```python
from build123d import *

# Parameters (mm, degrees)
SKETCH_1_W          = 100
SKETCH_1_H          = 75
EXTRUDE_1_DEPTH     = 3
SKETCH_2_R          = 2.5
CUT_EXTRUDE_1_DEPTH = 3
SKETCH_3_R          = 2.5
CUT_EXTRUDE_2_DEPTH = 3
EXTRUDE_2_DEPTH     = 3
FILLET_1_R          = 1.5


with BuildPart() as part:
    # 草图1 → 凸台-拉伸1 (new body)
    with BuildSketch(Plane(origin=(0, 0, 0), x_dir=(1, 0, 0), z_dir=(0, 1, 0))):
        Rectangle(SKETCH_1_W, SKETCH_1_H)
    extrude(amount=EXTRUDE_1_DEPTH)

    # 草图2 → 切除-拉伸1 (cut)
    with BuildSketch(Plane(origin=(0, 3, 0), x_dir=(1, 0, 0), z_dir=(0, 1, 0))):
        with Locations(Location((-46.9, 17.87, 0), (0, 0, 270))):
            Circle(SKETCH_2_R)
        with Locations(Location((-46.9, -31.338, 0), (0, 0, 90))):
            Circle(SKETCH_2_R)
        with Locations(Location((40.184, -31.338, 0), (0, 0, 270))):
            Circle(SKETCH_2_R)
        with Locations(Location((40.184, 17.87, 0), (0, 0, 90))):
            Circle(SKETCH_2_R)
    extrude(amount=-CUT_EXTRUDE_1_DEPTH, mode=Mode.SUBTRACT)

    # 草图3 → 切除-拉伸2 (cut)
    with BuildSketch(Plane(origin=(0, 3, 0), x_dir=(1, 0, 0), z_dir=(0, 1, 0))):
        with Locations(Location((-24, 25, 0), (0, 0, 270))):
            Circle(SKETCH_3_R)
        with Locations(Location((24, 25, 0), (0, 0, 90))):
            Circle(SKETCH_3_R)
        with Locations(Location((24, -25, 0), (0, 0, 270))):
            Circle(SKETCH_3_R)
        with Locations(Location((-24, -25, 0), (0, 0, 90))):
            Circle(SKETCH_3_R)
        with Locations(Location((0, 5, 0), (0, 0, 270))):
            Circle(SKETCH_3_R)
        with Locations(Location((0, 15, 0), (0, 0, 270))):
            Circle(SKETCH_3_R)
        with Locations(Location((0, -15, 0), (0, 0, 90))):
            Circle(SKETCH_3_R)
        with Locations(Location((0, -5, 0), (0, 0, 90))):
            Circle(SKETCH_3_R)
        with Locations(Location((10, 5, 0), (0, 0, 270))):
            Circle(SKETCH_3_R)
        with Locations(Location((10, 15, 0), (0, 0, 270))):
            Circle(SKETCH_3_R)
        with Locations(Location((10, -15, 0), (0, 0, 90))):
            Circle(SKETCH_3_R)
        with Locations(Location((10, -5, 0), (0, 0, 90))):
            Circle(SKETCH_3_R)
        with Locations(Location((20, 5, 0), (0, 0, 270))):
            Circle(SKETCH_3_R)
        with Locations(Location((20, 15, 0), (0, 0, 270))):
            Circle(SKETCH_3_R)
        with Locations(Location((20, -15, 0), (0, 0, 90))):
            Circle(SKETCH_3_R)
        with Locations(Location((20, -5, 0), (0, 0, 90))):
            Circle(SKETCH_3_R)
        with Locations(Location((-20, -5, 0), (0, 0, 270))):
            Circle(SKETCH_3_R)
        with Locations(Location((-20, -15, 0), (0, 0, 270))):
            Circle(SKETCH_3_R)
        with Locations(Location((-20, 15, 0), (0, 0, 90))):
            Circle(SKETCH_3_R)
        with Locations(Location((-20, 5, 0), (0, 0, 90))):
            Circle(SKETCH_3_R)
        with Locations(Location((-10, -5, 0), (0, 0, 270))):
            Circle(SKETCH_3_R)
        with Locations(Location((-10, -15, 0), (0, 0, 270))):
            Circle(SKETCH_3_R)
        with Locations(Location((-10, 15, 0), (0, 0, 90))):
            Circle(SKETCH_3_R)
        with Locations(Location((-10, 5, 0), (0, 0, 90))):
            Circle(SKETCH_3_R)
        with BuildLine():
            Line((-31.51322225, 8.5), (-31.51322225, -8.5))
            ThreePointArc((-31.51322225, -8.5), (-36.01322225, -13), (-40.51322225, -8.5))
            Line((-40.51322225, -8.5), (-40.51322225, 8.5))
            ThreePointArc((-40.51322225, 8.5), (-36.01322225, 13), (-31.51322225, 8.5))
        make_face()
        with BuildLine():
            Line((31.51322225, 8.5), (31.51322225, -8.5))
            ThreePointArc((31.51322225, -8.5), (36.01322225, -13), (40.51322225, -8.5))
            Line((40.51322225, -8.5), (40.51322225, 8.5))
            ThreePointArc((40.51322225, 8.5), (36.01322225, 13), (31.51322225, 8.5))
        make_face()
    extrude(amount=-CUT_EXTRUDE_2_DEPTH, mode=Mode.SUBTRACT)

    # 草图4 → 凸台-拉伸2 (add)
    with BuildSketch(Plane(origin=(0, 3, 0), x_dir=(1, 0, 0), z_dir=(0, 1, 0))):
        Polygon((-50, 22.87), (-51.2, 20.296591695), (-51.2, 15.443408305), (-50, 12.87), align=None)
        Polygon((-51.2, -28.911408305), (-50, -26.338), (-50, -36.338), (-51.2, -33.764591695), align=None)
    extrude(amount=-EXTRUDE_2_DEPTH)

    # 圆角1
    # the kernel refuses this fillet: 1.5 mm, written as the material it takes off along each edge
    with BuildSketch(Plane(origin=(50, -3.75, 37.5), x_dir=(0, 0, -1), z_dir=(0, 1, 0)), Plane(origin=(50, -3.75, -37.5), x_dir=(-1, 0, 0), z_dir=(0, 1, 0))) as fillet_1_piece_1:
        with BuildLine():
            CenterArc((FILLET_1_R, FILLET_1_R), FILLET_1_R, 180, 90)
            Line((0, FILLET_1_R), (-FILLET_1_R * 0.02, FILLET_1_R))
            Line((-FILLET_1_R * 0.02, FILLET_1_R), (-FILLET_1_R * 0.02, -FILLET_1_R * 0.02))
            Line((-FILLET_1_R * 0.02, -FILLET_1_R * 0.02), (FILLET_1_R, -FILLET_1_R * 0.02))
            Line((FILLET_1_R, -FILLET_1_R * 0.02), (FILLET_1_R, 0))
        make_face()
    extrude(amount=10.5, mode=Mode.SUBTRACT)
    with BuildSketch(Plane(origin=(-50, -3.653556486, 37.5), x_dir=(1, 0, 0), z_dir=(0, 1, 0))) as fillet_1_piece_2:
        with BuildLine():
            CenterArc((1.461422595, 1.5), FILLET_1_R, 193.02248013, 76.97751987)
            Line((0, 1.162), (-0.029228452, 1.15524))
            ThreePointArc((-0.029228452, 1.15524), (-0.03, 0.581), (-0.03, 0))
            Line((-0.03, 0), (0, -0.03))
            Line((0, -0.03), (1.461422595, -0.03))
            Line((1.461422595, -0.03), (1.461422595, 0))
        make_face()
    extrude(amount=10.307112973, mode=Mode.SUBTRACT)
    with BuildSketch(Plane(origin=(-50, -3.75, -37.5), x_dir=(1, 0, 0), z_dir=(0, 1, 0))) as fillet_1_piece_3:
        with BuildLine():
            CenterArc((FILLET_1_R, -FILLET_1_R), FILLET_1_R, 90, 90)
            Line((0, -FILLET_1_R), (-FILLET_1_R * 0.02, -FILLET_1_R))
            Line((-FILLET_1_R * 0.02, -FILLET_1_R), (-FILLET_1_R * 0.02, FILLET_1_R * 0.02))
            Line((-FILLET_1_R * 0.02, FILLET_1_R * 0.02), (FILLET_1_R, FILLET_1_R * 0.02))
            Line((FILLET_1_R, FILLET_1_R * 0.02), (FILLET_1_R, 0))
        make_face()
    extrude(amount=10.5, mode=Mode.SUBTRACT)


solid = part.part
```
Design review of the part built by this model. Coordinates are the model's own, in mm. A direction names the side the tool comes from. Round coordinates to 2 decimals unless told otherwise and drop trailing zeros. Write each loop counter-clockwise with the first axis right and the second up, starting at its lowest first coordinate (ties: lowest second). Pieces come first, ordered by that corner, then holes. Notation, with made-up numbers: (-7.75, 40) -> (18.25, 40) arc R31 cw to (18.25, 75) -> close; hole circle Ø7 at (-14.5, 21). An arc over 180 degrees is marked (long way). Write item = value, one per line. Start each with the question number.
1) Tool access review of faces 1 (the face through (36, 2, 13)), 2 (the face through (-50.59, 1.52, 35.07)), 3 (the face through (-50.608, 1.521, -14.175)): name each direction out of +Z, -Z, +X, -X, +Y, -Y from which nothing blocks a thin tool from reaching the whole face with its end or side.
2) Take a section at A-A, the plane x = -20. State the section outline as (y, z) points, plus the area to 3 significant figures.
3) Take a section at B-B, the plane z = 5. Count the separate pieces of the cut face and the enclosed holes in it, plus the area to 3 significant figures.
4) Take a section at C-C, the plane x = 24. State the section outline as (y, z) points, plus the area to 3 significant figures.
5) Take a section at D-D, the plane z = -25. State the section outline as (x, y) points.
6) Wall thickness on probe 1 along X at (y, z) = (2.1, -1.5); probe 2 along X at (y, z) = (2.35, 32); probe 3 along X at (y, z) = (1.5, 15.5): over which ranges is each line inside the solid? List them lowest first. Write a range as from..to.
7) Mouldability with a two-part tool opening along Z and no side actions: class faces 4 (the face through (-1, 0, -1)), 5 (the face through (17.89, 1.52, 3.66)), 6 (the face through (-1, 1, 37.5)) as +Z half, -Z half, draft (parallel to the pull), parting line (faces both ways), or undercut.
Results list:
q1.face_1 = +Y, -Y
q1.face_2 = +Z, -X, +Y, -Y
q1.face_3 = -X, +Y, -Y
q2.outline = (0, -37.5) -> (3, -37.5) -> (3, -17.5) -> (0, -17.5) -> close; (0, -12.5) -> (3, -12.5) -> (3, -7.5) -> (0, -7.5) -> close; (0, -2.5) -> (3, -2.5) -> (3, 2.5) -> (0, 2.5) -> close; (0, 7.5) -> (3, 7.5) -> (3, 12.5) -> (0, 12.5) -> close; (0, 17.5) -> (3, 17.5) -> (3, 37.5) -> (0, 37.5) -> close
q2.area = 165 mm²
q3.separate_pieces = 8
q3.enclosed_holes = 0
q3.area = 171 mm²
q4.outline = (0, -37.5) -> (3, -37.5) -> (3, -27.5) -> (0, -27.5) -> close; (0, -22.5) -> (3, -22.5) -> (3, 22.5) -> (0, 22.5) -> close; (0, 27.5) -> (3, 27.5) -> (3, 37.5) -> (0, 37.5) -> close
q4.area = 195 mm²
q5.outline = (-50, 0) -> (-26.5, 0) -> (-26.5, 3) -> (-50, 3) -> close; (-21.5, 0) -> (21.5, 0) -> (21.5, 3) -> (-21.5, 3) -> close; (26.5, 0) -> (50, 0) -> (50, 3) -> (26.5, 3) -> close
q6.probe_1 = -50..-40.51, -31.51..31.51, 40.51..50
q6.probe_2 = -51.2..-49.31, -44.49..37.77, 42.59..50
q6.probe_3 = -50..-22.45, -17.55..-12.45, -7.55..-2.45, 2.45..7.55, 12.45..17.55, 22.45..50
q7.face_4 = draft
q7.face_5 = undercut
q7.face_6 = +Z half
